from build123d import *

# Parameters (mm, degrees)
F0_W     = 457.2
F0_H     = 50.8
F1_DEPTH = 50.8
F2_W     = 50.8
F2_H     = 50.8
F3_DEPTH = 914.4
F4_W     = 50.8
F4_H     = 50.8
F5_DEPTH = 914.4
F6_W     = 50.8
F6_H     = 50.8
F7_DEPTH = 304.8
F8_R     = 7.9375
F9_DEPTH = 50.8


with BuildPart() as f1:
    # F0 (on Top) → F1 (new body)
    with BuildSketch(Plane.XY):
        Polygon((0, 2082.8), (0, 2133.6), (-50.8, 2133.6), (-50.8, 2082.8), (-50.8, 0), (0, 0), align=None)
        with Locations((228.6, 2108.2)):
            Rectangle(F0_W, F0_H)
        with Locations((-279.4, 2108.2)):
            Rectangle(F0_W, F0_H)
    extrude(amount=F1_DEPTH)

    # F2 (on face) → F3 (join)
    with BuildSketch(Plane.XY.offset(50.8)):
        with Locations((-482.6, 2108.2)):
            Rectangle(F2_W, F2_H)
        with Locations((431.8, 2108.2)):
            Rectangle(F2_W, F2_H)
    extrude(amount=F3_DEPTH)

    # F4 (on face) → F5 (join)
    with BuildSketch(Plane.XY.offset(50.8)):
        with Locations((-25.4, 1193.8)):
            Rectangle(F4_W, F4_H)
    extrude(amount=F5_DEPTH)

    # F6 (on face) → F7 (join)
    with BuildSketch(Plane.XY.offset(50.8)):
        with Locations((-25.4, 787.4)):
            Rectangle(F6_W, F6_H)
    extrude(amount=F7_DEPTH)

    # F8 (on face) → F9 (cut)
    with BuildSketch(Plane(origin=(-50.8, 0, 0), x_dir=(0, -1, 0), z_dir=(-1, 0, 0))):
        with Locations((-139.7, 25.4)):
            Circle(F8_R)
        with Locations((-38.1, 25.4)):
            Circle(F8_R)
    extrude(amount=-F9_DEPTH, mode=Mode.SUBTRACT)


solid = f1.part
Could you check a few things on this model? Use its own coordinates, in mm. A direction names the side the tool comes from. Coordinates: 2 decimals unless noted, no trailing zeros. Loops run counter-clockwise (first coordinate to the right, second up) from the corner with the lowest first, then second, coordinate; pieces in that order, holes last.
1. Imagine slicing it at A-A (z = 734). Please give me the cut outline in (x, y), and give its area (3 significant figures).
2. For faces 1 (the face through (-26, 993, 50.8)), 2 (the face through (0, 1191, 230)), 3 (the face through (-50.8, 1201, 266)), which set-ups out of +Z, -Z, +X, -X, +Y, -Y let a thin tool reach every point of the face, with its end or its side?
3. For P1, Ø15, axis at x = -20, z = 486, coming from the -Y side; P2, Ø2, axis at x = -45.5, y = 1066, coming from the +Z side; P3, Ø8, axis at x = -23, z = 100.5, coming from the -Y side, each with a flat end and sliding along its axis, tell me the tip position at first contact or that it passes through.
4. Imagine slicing it at B-B (z = 184.5). Please give me the cut outline in (x, y), and give its area (3 significant figures).
5. Imagine slicing it at C-C (y = 559). Please give me the cut outline in (x, z), and give its area (3 significant figures).
6. I need wall thicknesses on L1, parallel to Y at x = -26, z = 25; L2, parallel to Z at x = -34, y = 139.7; L3, parallel to Y at x = -40, z = 148. Which ranges of each line are inside material? Lowest first, please.
7. We'd pull the mould along Y, two halves only. Please class faces 4 (the face through (-26, 0, 25)), 5 (the face through (431, 2109, 965.2)), 6 (the face through (-26, 812.8, 201)): released by +Y, released by -Y, zero draft, split by the parting line, or undercut.
8. Imagine slicing it at D-D (x = 21). Please give me the cut outline in (y, z).
Computed values:
1. outline: (-508, 2082.8) - (-457.2, 2082.8) - (-457.2, 2133.6) - (-508, 2133.6) - close; (-50.8, 1168.4) - (0, 1168.4) - (0, 1219.2) - (-50.8, 1219.2) - close; (406.4, 2082.8) - (457.2, 2082.8) - (457.2, 2133.6) - (406.4, 2133.6) - close
1. area: 7,740 mm2
2. face 1: +Z, +X, -X
2. face 2: +Z, -Z, +X, -Y
2. face 3: +Z, -Z, -X, -Y
3. P1: stops at y = 1168.4
3. P2: stops at z = 50.8
3. P3: stops at y = 762
4. outline: (-508, 2082.8) - (-457.2, 2082.8) - (-457.2, 2133.6) - (-508, 2133.6) - close; (-50.8, 762) - (0, 762) - (0, 812.8) - (-50.8, 812.8) - close; (-50.8, 1168.4) - (0, 1168.4) - (0, 1219.2) - (-50.8, 1219.2) - close; (406.4, 2082.8) - (457.2, 2082.8) - (457.2, 2133.6) - (406.4, 2133.6) - close
4. area: 10,300 mm2
5. outline: (-50.8, 0) - (0, 0) - (0, 50.8) - (-50.8, 50.8) - close
5. area: 2,580 mm2
6. L1: y = 0 to 30.17, 46.03 to 131.77, 147.63 to 2133.6
6. L2: z = 0 to 17.46, 33.34 to 50.8
6. L3: y = 762 to 812.8, 1168.4 to 1219.2
7. face 4: released by -Y
7. face 5: zero draft
7. face 6: undercut
8. outline: (2082.8, 0) - (2133.6, 0) - (2133.6, 50.8) - (2082.8, 50.8) - close
